```python
from build123d import *

# Parameters (mm, degrees)
BOSS_EXTRUDE1_DEPTH      = 23
BOSS_EXTRUDE2_DEPTH      = 54
BOSS_EXTRUDE3_DEPTH      = 23
CUT_EXTRUDE1_DEPTH       = 12
CHAMFER1_SIZE            = 1
CHAMFER1_OF_MIRROR2_SIZE = 1
SKETCH7_W                = 28
SKETCH7_H                = 28
CUT_EXTRUDE2_DEPTH       = 10
F_12_0MM_DOWEL_HOLE1_D   = 12
CUT_EXTRUDE3_START       = 1.999999915
CUT_EXTRUDE3_DEPTH       = 36.000000085
CUT_EXTRUDE3_START_2     = -5
CUT_EXTRUDE3_2_DEPTH     = 10
CHAMFER2_START           = -23
CHAMFER2_2_DEPTH         = 46


with BuildPart() as part:
    # Sketch2 → Boss-Extrude1 (new, symmetric)
    with BuildSketch(Plane.XY):
        Polygon((99.985564599, 0), (-99.985564599, 0), (-104, -14), (-97.5, -14), (-97.5, -12.082323829), (97.5, -12.082323829), (97.5, -14), (104, -14), align=None)
    extrude(amount=BOSS_EXTRUDE1_DEPTH, both=True)

    # Sketch3 → Boss-Extrude2 (add)
    with BuildSketch(Plane(origin=(0, 0, 0), x_dir=(1, 0, 0), z_dir=(0, 1, 0))):
        with BuildLine():
            Line((48.856934001, -23), (28, -23))
            Line((28, -23), (28, 23))
            Line((28, 23), (48.856934001, 23))
            ThreePointArc((48.856934001, 23), (54, 0), (48.856934001, -23))
        make_face()
    boss_extrude2 = extrude(amount=BOSS_EXTRUDE2_DEPTH)

    # Mirror1: Boss-Extrude2 across plane
    add(boss_extrude2.mirror(Plane(origin=(0, 0, 0), x_dir=(0, 0, 1), z_dir=(1, 0, 0))))

    # Sketch4 → Boss-Extrude3 (add, symmetric)
    with BuildSketch(Plane.XY):
        with BuildLine():
            Line((-28, 38), (-23.664319132, 38))
            ThreePointArc((-23.664319132, 38), (0, 10), (23.664319132, 38))
            Line((23.664319132, 38), (28, 38))
            Line((28, 38), (28, 0))
            Line((28, 0), (-28, 0))
            Line((-28, 0), (-28, 38))
        make_face()
    extrude(amount=BOSS_EXTRUDE3_DEPTH, both=True)

    # Sketch5 → Cut-Extrude1 (cut)
    with BuildSketch(Plane(origin=(0, 0, 0), x_dir=(1, 0, 0), z_dir=(0, 1, 0))):
        with BuildLine():
            Line((-81, 6), (-73, 6))
            ThreePointArc((-73, 6), (-67, 0), (-73, -6))
            Line((-73, -6), (-81, -6))
            ThreePointArc((-81, -6), (-87, 0), (-81, 6))
        make_face()
    cut_extrude1 = extrude(amount=-CUT_EXTRUDE1_DEPTH, mode=Mode.SUBTRACT)

    # Chamfer1
    chamfer1_edges = [part.edges().sort_by_distance(p)[0] for p in [
        (-87, 0, 0),
        (-77, 0, 6),
        (-67, 0, 0),
        (-77, 0, -6),
    ]]
    chamfer(chamfer1_edges, length=CHAMFER1_SIZE)

    # Mirror2: Cut-Extrude1 across plane
    add(cut_extrude1.mirror(Plane(origin=(0, 0, 0), x_dir=(0, 0, 1), z_dir=(1, 0, 0))), mode=Mode.SUBTRACT)

    # Chamfer1 of Mirror2
    chamfer1_of_mirror2_edges = [part.edges().sort_by_distance(p)[0] for p in [
        (87, 0, 0),
        (77, 0, 6),
        (67, 0, 0),
        (77, 0, -6),
    ]]
    chamfer(chamfer1_of_mirror2_edges, length=CHAMFER1_OF_MIRROR2_SIZE)

    # Sketch7 → Cut-Extrude2 (cut)
    with BuildSketch(Plane.XZ.offset(12.082323829)):
        with Locations((-39, 0)):
            Rectangle(SKETCH7_W, SKETCH7_H)
    cut_extrude2 = extrude(amount=-CUT_EXTRUDE2_DEPTH, mode=Mode.SUBTRACT)

    # Mirror3: Cut-Extrude2 across plane
    add(cut_extrude2.mirror(Plane(origin=(0, 0, 0), x_dir=(0, 0, 1), z_dir=(1, 0, 0))), mode=Mode.SUBTRACT)

    # Ø12.0mm Dowel Hole1 (through all)
    with Locations(Plane(origin=(0, -2.082323829, 0), x_dir=(-1, 0, 0), z_dir=(0, -1, 0))):
        with Locations((39, 0), (-39, 0)):
            Hole(F_12_0MM_DOWEL_HOLE1_D / 2)

    # Cut-Extrude3: read off the stored shape, not the designer's step
    # Cut-Extrude3 outline → Cut-Extrude3 (cut)
    with BuildSketch(Plane(origin=(0, 0, 0), x_dir=(1, 0, 0), z_dir=(0, 1, 0)).offset(CUT_EXTRUDE3_START)):
        with BuildLine():
            add(Edge.make_bspline(
                [(4, 0), (4, 1.059018663), (3.564754015, 2.092267125), (2.091459192, 3.565228094), (1.047779124, 3.999399314), (-1.043187737, 4.000599369), (-2.08248981, 3.57393755), (-3.572744195, 2.08453648), (-3.999590121, 1.046654427), (-4.000409264, -1.043519212), (-3.567812098, -2.087662609), (-2.094321457, -3.563907402), (-1.060428453, -3.999150693), (1.054011474, -4.000846733), (2.089559005, -3.5661873), (3.563043078, -2.094915922), (4, -1.059018663), (4, 0)],
                knots=[0, 0, 0, 0, 0.125, 0.125, 0.25, 0.25, 0.375, 0.375, 0.5, 0.5, 0.625, 0.625, 0.75, 0.75, 0.875, 0.875, 1, 1, 1, 1], degree=3))
        make_face()
    extrude(amount=CUT_EXTRUDE3_DEPTH, mode=Mode.SUBTRACT)

    # Cut-Extrude3 2 outline → Cut-Extrude3 2 (add)
    with BuildSketch(Plane.XY.offset(CUT_EXTRUDE3_START_2)):
        with BuildLine():
            Line((5, 2.504711719), (4, 2.335680868))
            ThreePointArc((4, 2.335680868), (2.007030354, 2.084067462), (2.16e-07, 2))
            Line((2.16e-07, 2), (5, 1.999999915))
            Line((5, 1.999999915), (5, 2.504711719))
        make_face()
        with BuildLine():
            Line((-5, 1.999999915), (2.16e-07, 2))
            ThreePointArc((2.16e-07, 2), (-2.014229388, 2.084672698), (-4.014246469, 2.338093372))
            Line((-4.014246469, 2.338093372), (-5, 2.505326626))
            Line((-5, 2.505326626), (-5, 1.999999915))
        make_face()
    extrude(amount=CUT_EXTRUDE3_2_DEPTH)

    # Chamfer2: read off the stored shape, not the designer's step
    # Chamfer2 outline → Chamfer2 (revolve, cut)
    with BuildSketch(Plane.XZ.offset(-34)):
        Polygon((24, 23), (24, 21), (26, 23), align=None)
        Polygon((26, -23), (24, -21), (24, -23), align=None)
    revolve(axis=Axis((0, 34, 0), (0, 0, 1)), mode=Mode.SUBTRACT)

    # Chamfer2 2 outline → Chamfer2 2 (cut)
    with BuildSketch(Plane.XY.offset(CHAMFER2_START)):
        with BuildLine():
            ThreePointArc((23.664319132, 38), (23.796597884, 37.118000823), (23.896015012, 36.231695881))
            Line((23.896015012, 36.231695881), (25.664319132, 38))
            Line((25.664319132, 38), (23.664319132, 38))
        make_face()
        with BuildLine():
            Line((-25.399406115, 38), (-23.922856044, 35.922747689))
            ThreePointArc((-23.922856044, 35.922747689), (-23.816245603, 36.964193884), (-23.664319132, 38))
            Line((-23.664319132, 38), (-25.399406115, 38))
        make_face()
    extrude(amount=CHAMFER2_2_DEPTH, mode=Mode.SUBTRACT)


solid = part.part
```
The listing builds one solid part. Answer for the finished solid, in the listing's coordinates (mm). A direction names the side the tool comes from. Round coordinates to 2 decimals unless told otherwise and drop trailing zeros. Loops run counter-clockwise (first coordinate to the right, second up) from the corner with the lowest first, then second, coordinate; pieces in that order, holes last.
1) Given P1, Ø3, axis at y = -7.5, z = 1.5, coming from the +X side; P2, Ø6, axis at x = -24.5, z = -15, coming from the -Y side; P3, Ø0.7, axis at x = 27, z = 8.5, coming from the +Y side, each flat-ended and moving along its own axis, determine where each tip first touches the part or whether it passes through.
Outcome:
P1: stops at x = 102.57
P2: stops at y = -12.08
P3: stops at y = 38
2) A cutting plane is placed at A-A on x = -39. Determine the outline of the cut face in (y, z).
Outcome:
outline: (-12.08, -23) - (54, -23) - (54, -6) - (-2.08, -6) - (-2.08, -14) - (-12.08, -14) - close; (-12.08, 14) - (-2.08, 14) - (-2.08, 6) - (54, 6) - (54, 23) - (-12.08, 23) - close
3) For faces 5 (the face through (-45.4, -2.082, 0.2)), 6 (the face through (102.02, -7.1, 0.32)), 7 (the face through (66.8, -0.8, -0.1)), 8 (the face through (-1, -12.082, 0)), 9 (the face through (44, 54, 5)), determine the directions among +Z, -Z, +X, -X, +Y, -Y from which every point of the face is accessible in a straight line to the end or side of a thin tool.
Outcome:
face 5: -Y
face 6: +Z, -Z, +X, +Y
face 7: +Y
face 8: +Z, -Z, -Y
face 9: +Z, -Z, +X, -X, +Y
4) A cutting plane is placed at C-C on z = 0. Give the number of separate pieces and of enclosed holes in the cut face, plus the area to 3 significant figures.
Outcome:
separate pieces: 3
enclosed holes: 0
area: 3,870 mm2
5) For a pull along Z with two mould halves and no side action, classify faces 1 (the face through (-87, -6, 0)), 2 (the face through (54, 27, 0)), 3 (the face through (-25, -7, 0)), 4 (the face through (75, 0, 11)) as released by +Z, released by -Z, zero draft, split by the parting line, or undercut.
Outcome:
face 1: undercut
face 2: split by the parting line
face 3: undercut
face 4: zero draft
6) A cutting plane is placed at B-B on y = -6. Determine the outline of the cut face in (x, z), plus the area to 3 significant figures.
Outcome:
outline: (-101.71, -23) - (101.71, -23) - (101.71, 23) - (-101.71, 23) - close; hole (-81, -6) - (-73, -6) arc R6 ccw to (-73, 6) - (-81, 6) arc R6 ccw to start; hole (-53, -14) - (-25, -14) - (-25, 14) - (-53, 14) - close; hole (25, -14) - (53, -14) - (53, 14) - (25, 14) - close; hole (73, -6) - (81, -6) arc R6 ccw to (81, 6) - (73, 6) arc R6 ccw to start
area: 7,370 mm2
7) Consider line 1 (Z direction, x = 33, y = -3); line 2 (Z direction, x = -39, y = 9); line 3 (X direction, y = 50.5, z = 10.5). Determine where each line is inside the solid, lowest interval first.
Outcome:
line 1: z = -23 to -14, 14 to 23
line 2: z = -23 to -6, 6 to 23
line 3: x = -52.97 to -28, 28 to 52.97
